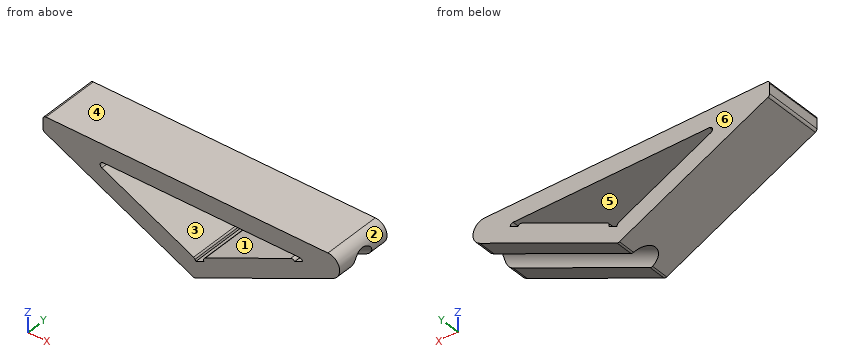
```python
from build123d import *

# Parameters (mm, degrees)
F1_DEPTH  = 50
F3_R      = 1
F4_R      = 4
F5_R      = 4
F6_DEPTH  = 116.6842043143
F8_DEPTH  = 50.0010001
F9_R      = 0.99999
F10_DEPTH = 30


# Not quite as in the source:
# - a fillet or chamfer is up to 0.001 mm smaller than in the source, because OpenCascade refuses the exact size


with BuildPart() as f1:
    # F0 (on Front) → F1 (new body)
    with BuildSketch(Plane.XZ):
        Polygon((-63.4415450926, -29.5832783218), (0, 0), (-115, 0), (-115, -5), align=None)
    extrude(amount=F1_DEPTH)

    # F3
    f3_edges = [f1.edges().sort_by_distance(p)[0] for p in [
        (-63.441545, -25, -29.583278),
        (-115, -25, -5),
        (-115, -25, 0),
    ]]
    fillet(f3_edges, radius=F3_R)

    # F4
    f4_edges = [f1.edges().sort_by_distance(p)[0] for p in [
        (0, -25, 0),
    ]]
    fillet(f4_edges, radius=F4_R)

    # F5 (on face) → F6 (cut, through all)
    with BuildSketch(Plane(origin=(0, 0, 0), x_dir=(0, 1, 0), z_dir=(0.906307787, 0, 0.4226182617))):
        with Locations((-40, 0)):
            Circle(F5_R)
    extrude(amount=-F6_DEPTH, mode=Mode.SUBTRACT)

    # F7 (on Front) → F8 (cut, through all)
    with BuildSketch(Plane.XZ):
        Polygon((-27.064251022, -6), (-98.9616948614, -6), (-63.4130640807, -22.9497298941), (-62.990445819, -23.8560376812), (-60.2715224579, -22.588182896), (-60.6941407196, -21.6818751089), (-29.7831743831, -7.2678547852), (-29.3605561213, -8.1741625723), (-26.6416327602, -6.906307787), align=None)
    extrude(amount=F8_DEPTH, mode=Mode.SUBTRACT)

    # F9 (radius 1 in the source; OpenCascade refuses exactly that, so slightly less here)
    f9_edges = [f1.edges().sort_by_distance(p)[0] for p in [
        (-98.961695, -25, -6),
        (-60.694141, -25, -21.681875),
        (-29.783174, -25, -7.267855),
        (-27.064251, -25, -6),
        (-63.413064, -25, -22.94973),
    ]]
    fillet(f9_edges, radius=F9_R)

    # F0 (on Front) → F10 (cut)
    with BuildSketch(Plane.XZ):
        Polygon((-63.4415450926, -29.5832783218), (0, 0), (-115, 0), (-115, -5), align=None)
    extrude(amount=F10_DEPTH, mode=Mode.SUBTRACT)


solid = f1.part
```
Here's how the part is built. I have some questions about the finished solid (model axes, mm). Face numbers are marked on the shaded views. A direction names the side the tool comes from. Coordinates: 2 decimals unless noted, no trailing zeros. Loops run counter-clockwise (first coordinate to the right, second up) from the corner with the lowest first, then second, coordinate; pieces in that order, holes last. Notation, with made-up numbers: (-0.75, 51.25) - (51.25, 51.25) arc R16 ccw to (51.25, 62.25) - close; hole circle Ø2 at (-5, 45). An arc over 180 degrees is marked (long way). Answer as CSV lines item,"result".
Q1. For the marked faces 5 and 6, which set-ups out of +Z, -Z, +X, -X, +Y, -Y let a thin tool reach every point of the face, with its end or its side?
Response:
face 5,"+Y, -Y"
face 6,"+Z, -Z, +X, -X, +Y"
Q2. If we section it at B-B, the plane x = -93: Write out the boundary of the cut face in (y, z), and give its area (3 significant figures).
Response:
outline,"(-50, -15.49) - (-30, -15.49) - (-30, -8.84) - (-50, -8.84) - close; (-50, -6) - (-30, -6) - (-30, 0) - (-50, 0) - close"
area,"253 mm2"
Q3. We'd pull the mould along X, two halves only. Please class the marked faces 1, 2, 3 and 4: pulls with the +X half, pulls with the -X half, needs draft (parallel to the pull), parting line crosses it, or undercut.
Response:
face 1,"undercut"
face 2,"pulls with the +X half"
face 3,"undercut"
face 4,"needs draft"
Q4. For pin 1 (5 mm diameter, centred on y = -47, z = -5.5, fed in from +X); pin 2 (1 mm diameter, centred on x = -64.5, y = -38.5, fed in from -Z); pin 3 (1 mm diameter, centred on x = -100, y = -42.5, fed in from -Z); pin 4 (8 mm diameter, centred on y = -43, z = -21, fed in from -X), each with a flat end and sliding along its axis, tell me the tip position at first contact or that it passes through.
Response:
pin 1,"x = -14.04"
pin 2,"z = -26.33"
pin 3,"z = -12.39"
pin 4,"x = -89.83"
Q5. If I drill on L1, parallel to X at y = -46.25, z = -9.25; L2, parallel to Z at x = -43.5, y = -35; L3, parallel to Z at x = -24.5, y = -42, over which ranges is the centre line in solid material (lowest first)? Write a range as [from, to].
Response:
L1,"[-106.09, -92.15], [-34.03, -19.84]"
L2,"[-20.28, -13.66], [-6, 0]"
L3,"[-7.6, 0]"
